Input: part model. Units: mm. Frame: model coordinates. Round coordinates to 2 decimals unless told otherwise and drop trailing zeros. Order: outer loops, then holes, each group sorted by start corner. A loop starts at its lowest first (then second) coordinate and runs counter-clockwise, first axis right, second up. Notation, with made-up numbers: (-17, -23.75) -> (20, -23.75) arc R25 ccw to (20, -9.75) -> close; hole circle Ø2 at (-36.5, 14). An arc over 180 degrees is marked (long way). Use a Markdown table: item, result.
from build123d import *

# Parameters (mm, degrees)
F1_W     = 80
F1_H     = 1000
F2_DEPTH = 10
F3_R     = 10
F5_DEPTH = 10.001


with BuildPart() as f2:
    # F1 (on Front) → F2 (new body)
    with BuildSketch(Plane.XZ):
        Rectangle(F1_W, F1_H)
    extrude(amount=F2_DEPTH)

    # F3
    f3_edges = [f2.edges().sort_by_distance(p)[0] for p in [
        (40, -5, -500),
        (-40, -5, -500),
    ]]
    fillet(f3_edges, radius=F3_R)

    # F4 (on face) → F5 (cut, through all)
    with BuildSketch(Plane.XZ.offset(10)):
        with BuildLine():
            Line((-22.5166852265, -380), (22.5166852265, -380))
            ThreePointArc((22.5166852265, -380), (24.8737078304, -380.5904144816), (26.6740823229, -382.2222222222))
            ThreePointArc((26.6740823229, -382.2222222222), (33.5276684148, -381.8856180832), (30, -376))
            Line((30, -376), (30, -374))
            ThreePointArc((30, -374), (33.5276684148, -368.1143819168), (26.6740823229, -367.7777777778))
            ThreePointArc((26.6740823229, -367.7777777778), (24.8737078304, -369.4095855184), (22.5166852265, -370))
            Line((22.5166852265, -370), (-22.5166852265, -370))
            ThreePointArc((-22.5166852265, -370), (-24.8737078304, -369.4095855184), (-26.6740823229, -367.7777777778))
            ThreePointArc((-26.6740823229, -367.7777777778), (-33.5276684148, -368.1143819168), (-30, -374))
            Line((-30, -374), (-30, -376))
            ThreePointArc((-30, -376), (-33.5276684148, -381.8856180832), (-26.6740823229, -382.2222222222))
            ThreePointArc((-26.6740823229, -382.2222222222), (-24.8737078304, -380.5904144816), (-22.5166852265, -380))
        make_face()
        with BuildLine():
            Line((30, -126), (30, -124))
            ThreePointArc((30, -124), (33.5276684148, -118.1143819168), (26.6740823229, -117.7777777778))
            ThreePointArc((26.6740823229, -117.7777777778), (24.8737078304, -119.4095855184), (22.5166852265, -120))
            Line((22.5166852265, -120), (-22.5166852265, -120))
            ThreePointArc((-22.5166852265, -120), (-24.8737078304, -119.4095855184), (-26.6740823229, -117.7777777778))
            ThreePointArc((-26.6740823229, -117.7777777778), (-33.5276684148, -118.1143819168), (-30, -124))
            Line((-30, -124), (-30, -126))
            ThreePointArc((-30, -126), (-33.5276684148, -131.8856180832), (-26.6740823229, -132.2222222222))
            ThreePointArc((-26.6740823229, -132.2222222222), (-24.8737078304, -130.5904144816), (-22.5166852265, -130))
            Line((-22.5166852265, -130), (22.5166852265, -130))
            ThreePointArc((22.5166852265, -130), (24.8737078304, -130.5904144816), (26.6740823229, -132.2222222222))
            ThreePointArc((26.6740823229, -132.2222222222), (33.5276684148, -131.8856180832), (30, -126))
        make_face()
        with BuildLine():
            Line((30, 124), (30, 126))
            ThreePointArc((30, 126), (33.5276684148, 131.8856180832), (26.6740823229, 132.2222222222))
            ThreePointArc((26.6740823229, 132.2222222222), (24.8737078304, 130.5904144816), (22.5166852265, 130))
            Line((22.5166852265, 130), (-22.5166852265, 130))
            ThreePointArc((-22.5166852265, 130), (-24.8737078304, 130.5904144816), (-26.6740823229, 132.2222222222))
            ThreePointArc((-26.6740823229, 132.2222222222), (-33.5276684148, 131.8856180832), (-30, 126))
            Line((-30, 126), (-30, 124))
            ThreePointArc((-30, 124), (-33.5276684148, 118.1143819168), (-26.6740823229, 117.7777777778))
            ThreePointArc((-26.6740823229, 117.7777777778), (-24.8737078304, 119.4095855184), (-22.5166852265, 120))
            Line((-22.5166852265, 120), (22.5166852265, 120))
            ThreePointArc((22.5166852265, 120), (24.8737078304, 119.4095855184), (26.6740823229, 117.7777777778))
            ThreePointArc((26.6740823229, 117.7777777778), (33.5276684148, 118.1143819168), (30, 124))
        make_face()
        with BuildLine():
            Line((30, 374), (30, 376))
            ThreePointArc((30, 376), (33.5276684148, 381.8856180832), (26.6740823229, 382.2222222222))
            ThreePointArc((26.6740823229, 382.2222222222), (24.8737078304, 380.5904144816), (22.5166852265, 380))
            Line((22.5166852265, 380), (-22.5166852265, 380))
            ThreePointArc((-22.5166852265, 380), (-24.8737078304, 380.5904144816), (-26.6740823229, 382.2222222222))
            ThreePointArc((-26.6740823229, 382.2222222222), (-33.5276684148, 381.8856180832), (-30, 376))
            Line((-30, 376), (-30, 374))
            ThreePointArc((-30, 374), (-33.5276684148, 368.1143819168), (-26.6740823229, 367.7777777778))
            ThreePointArc((-26.6740823229, 367.7777777778), (-24.8737078304, 369.4095855184), (-22.5166852265, 370))
            Line((-22.5166852265, 370), (22.5166852265, 370))
            ThreePointArc((22.5166852265, 370), (24.8737078304, 369.4095855184), (26.6740823229, 367.7777777778))
            ThreePointArc((26.6740823229, 367.7777777778), (33.5276684148, 368.1143819168), (30, 374))
        make_face()
    extrude(amount=-F5_DEPTH, mode=Mode.SUBTRACT)


solid = f2.part
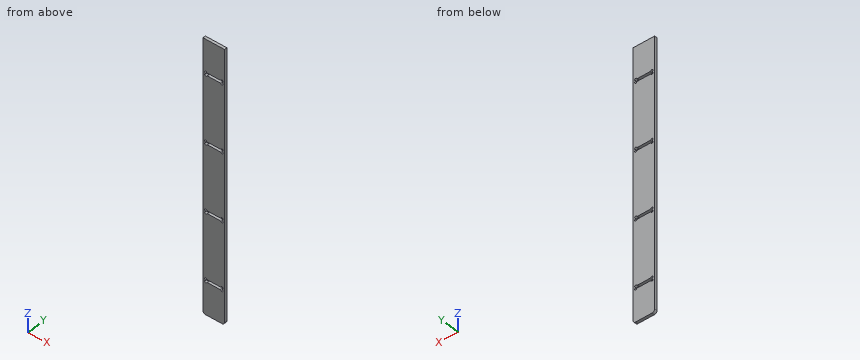
1) Cut plane A-A on x = -7. Return loops of the section in (y, z).
Answer key:
| item | result |
|---|---|
| outline | (-10, -500) -> (0, -500) -> (0, -380) -> (-10, -380) -> close; (-10, -370) -> (0, -370) -> (0, -130) -> (-10, -130) -> close; (-10, -120) -> (0, -120) -> (0, 120) -> (-10, 120) -> close; (-10, 130) -> (0, 130) -> (0, 370) -> (-10, 370) -> close; (-10, 380) -> (0, 380) -> (0, 500) -> (-10, 500) -> close |
2) Ray query, probe 1 along Z at (x, y) = (5.5, -4.5); probe 2 along Z at (x, y) = (29, -6.25). Return the intervals inside material, ascending.
Answer key:
| item | result |
|---|---|
| probe 1 | z = -500 to -380, -370 to -130, -120 to 120, 130 to 370, 380 to 500 |
| probe 2 | z = -500 to -383.87, -366.13 to -133.87, -116.13 to 116.13, 133.87 to 366.13, 383.87 to 500 |
3) Cut plane B-B on y = -6. State how many separate pieces and enclosed holes the cut face has, and give its area (3 significant figures).
Answer key:
| item | result |
|---|---|
| separate pieces | 1 |
| enclosed holes | 4 |
| area | 76,900 mm^2 |
